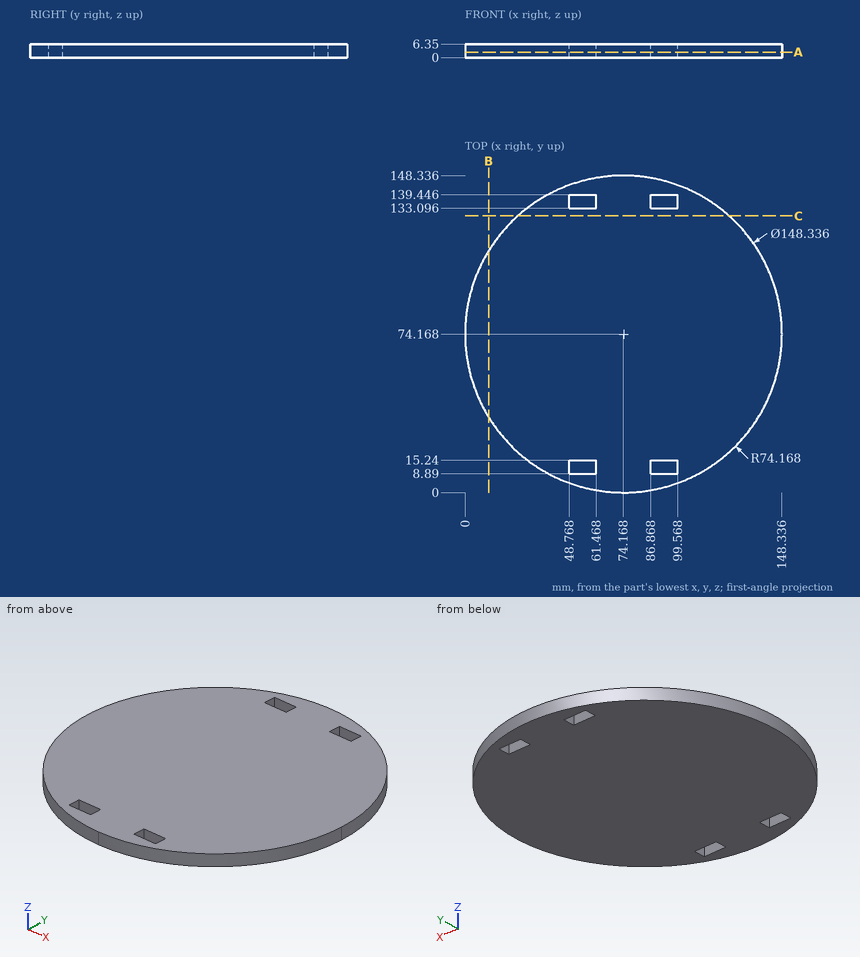
Job drawing, mm, ordinate dimensions from the low corner. One solid piece. Give positions to 0.01 mm unless a question says otherwise; leave off trailing zeros. Write each loop counter-clockwise with the first axis right and the second up, starting at its lowest first coordinate (ties: lowest second). Pieces come first, ordered by that corner, then holes. Notation, with made-up numbers: (29.25, 16) - (61.25, 16) arc R12 ccw to (61.25, 35) - close; hole circle Ø11 at (0, 23.25). An arc over 180 degrees is marked (long way). Use one line per item in the form item = value. Start each with the question number.
1. Probe line 1 (Y direction, x = 57.5, z = 3); line 2 (Y direction, x = 87, z = 4); line 3 (Y direction, x = 113, z = 4.5). List the from-to ranges inside material, lowest first. Write a range as [from, to].
2. Band-saw the part on C-C on y = 129.5. Write the cut outline in (x, z), plus the area to 3 significant figures.
3. Drop flat-ended pins along their axis: pin 1 Ø1.9 at (x, z) = (55, 3) entering from -Y; pin 2 Ø1.9 at (x, z) = (56, 3.5) entering from +Y; pin 3 Ø3 at (y, z) = (66, 1) entering from +X. Give the stop position or say it passes through.
4. Band-saw the part on B-B on x = 11. Write the cut outline in (y, z).
5. Band-saw the part on A-A on z = 2.5. Write the cut outline in (x, y), plus the area to 3 significant figures.
Conclusion:
q1.line_1 = [1.9, 8.89], [15.24, 133.1], [139.45, 146.44]
q1.line_2 = [1.12, 8.89], [15.24, 133.1], [139.45, 147.22]
q1.line_3 = [10.98, 137.36]
q2.outline = (24.78, 0) - (123.56, 0) - (123.56, 6.35) - (24.78, 6.35) - close
q2.area = 627 mm²
q3.pin_1 = 2.27
q3.pin_2 = 146.31
q3.pin_3 = 148.04
q4.outline = (35.3, 0) - (113.04, 0) - (113.04, 6.35) - (35.3, 6.35) - close
q5.outline = (74.17, 0) arc R74.17 ccw to (148.34, 74.17) arc R74.17 ccw (long way) to start; hole (48.77, 8.89) - (61.47, 8.89) - (61.47, 15.24) - (48.77, 15.24) - close; hole (48.77, 133.1) - (61.47, 133.1) - (61.47, 139.45) - (48.77, 139.45) - close; hole (86.87, 8.89) - (99.57, 8.89) - (99.57, 15.24) - (86.87, 15.24) - close; hole (86.87, 133.1) - (99.57, 133.1) - (99.57, 139.45) - (86.87, 139.45) - close
q5.area = 17,000 mm²
